Read the model definition and answer for the solid it produces. Units are mm, in the model's axes. A direction names the side the tool comes from. Give positions to 0.01 mm unless a question says otherwise; leave off trailing zeros. Order: outer loops, then holes, each group sorted by start corner. A loop starts at its lowest first (then second) coordinate and runs counter-clockwise, first axis right, second up. Notation, with made-up numbers: M 46,78.25 L 68,78.25 A14 ccw 68,96.25 Z; hole C -18.5,6 d8. An arc over 180 degrees is marked long. One line per item, written item: value.
from build123d import *

# Parameters (mm, degrees)
BOSS_EXTRUDE1_DEPTH = 20


with BuildPart() as part:
    # Sketch1 → Boss-Extrude1 (new body)
    with BuildSketch(Plane.XY):
        Polygon((65.303956044, 33.516483516), (-43.956043956, 33.516483516), (-47.956043956, 33.516483516), (-47.956043956, -66.483516484), (-43.956043956, -66.483516484), (-43.956043956, -51.483516484), (42.710622711, 13.516483516), (65.303956044, 13.516483516), align=None)
        Polygon((36.043956044, 13.516483516), (-43.956043956, -46.483516484), (-43.956043956, 13.516483516), align=None, mode=Mode.SUBTRACT)
    extrude(amount=BOSS_EXTRUDE1_DEPTH)


solid = part.part
1) Find section B-B, the plane z = 12.75. Write down the section's boundary in (x, y).
Reported:
outline: M -47.96,-66.48 L -43.96,-66.48 L -43.96,-51.48 L 42.71,13.52 L 65.3,13.52 L 65.3,33.52 L -47.96,33.52 Z; hole M -43.96,-46.48 L 36.04,13.52 L -43.96,13.52 Z
2) Determine the mould class of faces 4 (the face through (-5, 13.516, 10)), 5 (the face through (9, 33.516, 10)), 6 (the face through (0, 17, 0)) for opening direction Y: +Y half, -Y half, draft (parallel to the pull), parting line (faces both ways), or undercut.
Reported:
face 4: undercut
face 5: +Y half
face 6: draft
3) Each of these flat-tipped pins is pushed along its axis until it touches: pin 1 Ø6 at (x, z) = (53, 7) entering from -Y; pin 2 Ø1 at (y, z) = (-27.5, 14.5) entering from +X; pin 3 Ø6 at (y, z) = (-19.5, 15) entering from +X. Where does it stop, or does it pass through?
Reported:
pin 1: stops at y = 13.52
pin 2: stops at x = -11.31
pin 3: stops at x = 2.69
4) Find section A-A, the plane y = -29.5. Write down the section's boundary in (x, z), plus the area to 3 significant figures.
Reported:
outline: M -47.96,0 L -43.96,0 L -43.96,20 L -47.96,20 Z; M -21.31,0 L -14.64,0 L -14.64,20 L -21.31,20 Z
area: 213 mm^2
5) Find section D-D, the plane x = 51.5. Write down the section's boundary in (y, z), plus the area to 3 significant figures.
Reported:
outline: M 13.52,0 L 33.52,0 L 33.52,20 L 13.52,20 Z
area: 400 mm^2
6) Find section C-C, the plane x = -15. Write down the section's boundary in (y, z), plus the area to 3 significant figures.
Reported:
outline: M -29.77,0 L -24.77,0 L -24.77,20 L -29.77,20 Z; M 13.52,0 L 33.52,0 L 33.52,20 L 13.52,20 Z
area: 500 mm^2
7) Which of the six approach directions +Z, -Z, +X, -X, +Y, -Y give full straight-line access (tool end or side, diameter ignored) to faces 1 (the face through (-43.956, -59, 10)), 2 (the face through (-43.956, -17, 10)), 3 (the face through (0, 17, 20))?
Reported:
face 1: +Z, -Z, +X, -Y
face 2: +Z, -Z
face 3: +Z, +X, -X, +Y, -Y
8) Consider probe 1 along Y at (x, z) = (24, 11.5); probe 2 along Y at (x, z) = (-1.5, 12.75); probe 3 along X at (y, z) = (8, 2.25). Determine where each line is inside the solid, lowest interval first.
Reported:
probe 1: y = -0.52 to 4.48, 13.52 to 33.52
probe 2: y = -19.64 to -14.64, 13.52 to 33.52
probe 3: x = -47.96 to -43.96, 28.69 to 35.36
